Build history of the part. All positions in model axes, mm. A direction names the side the tool comes from. Round coordinates to 2 decimals unless told otherwise and drop trailing zeros. Order: outer loops, then holes, each group sorted by start corner. A loop starts at its lowest first (then second) coordinate and runs counter-clockwise, first axis right, second up. Notation, with made-up numbers: M 38,-24.5 L 62,-24.5 A35 ccw 62,13.5 Z; hole C 6.25,-17 d2. An arc over 180 degrees is marked long. One line per item, written item: value. Start each with the question number.
Item 1: Pin check, flat tips, straight feed: pin 1 (4 mm diameter, centred on y = -2.5, z = 9, fed in from -X); pin 2 (0.8 mm diameter, centred on y = 0, z = 1, fed in from -X); pin 3 (0.8 mm diameter, centred on y = 0, z = 0.5, fed in from +X). Stop position of each tip, or through.
Item 2: Band-saw the part on A-A, the plane z = 10.25. Write the cut outline in (x, y) (3 decimals), then the cut area to 3 significant figures.
Item 3: Band-saw the part on B-B, the plane x = 3. Write the cut outline in (y, z), then the cut area to 3 significant figures.
Item 4: Two-plate mould, pull along Y, no slides. Class faces 5 (the cylindrical face through (1.224, -0.507, 8.52)), 6 (the cylindrical face through (-2.686, -2.06, 2.73)), 7 (the flat face through (-1, -2, 9.78)): +Y half, -Y half, draft (parallel to the pull), parting line (faces both ways), or undercut.
Item 5: Tool access for faces 1 (the flat face through (0, 2.2, 2.35)), 2 (the cylindrical face through (-0.5, -2.4, 12.5)), 3 (the flat face through (0.4, 0, 1)), 4 (the cylindrical face through (0, -2, 6)): list every direction of +Z, -Z, +X, -X, +Y, -Y with a clear straight run to the whole face (end or side of a thin tool).
Item 6: Probe L1, parallel to X at y = 0, z = 8 (3 decimals); L2, parallel to Z at x = 1, y = 0.75; L3, parallel to X at y = 0, z = 11.25 (3 decimals). List the from-to ranges inside material, lowest first.
```python
from build123d import *

# Parameters (mm, degrees)
F0_R      = 3.385
F1_DEPTH  = 15.2
F2_R      = 3.385
F3_DEPTH  = 2.35
F4_DEPTH  = 1.65
F6_R      = 3.385
F6_R_2    = 2.45
F7_DEPTH  = 12.08
F9_R      = 3.385
F9_R_2    = 2
F10_DEPTH = 3
F11_R     = 2.45
F11_R_2   = 2
F12_DEPTH = 0.77
F31_R     = 1.325
F32_DEPTH = 13.55


with BuildPart() as f1:
    # F0 (on Top) → F1 (new body)
    with BuildSketch(Plane.XY):
        Circle(F0_R)
    extrude(amount=F1_DEPTH)

    # F2 (on face) → F3 (cut)
    with BuildSketch(Plane(origin=(0, 0, 0), x_dir=(1, 0, 0), z_dir=(0, 0, -1))):
        Circle(F2_R)
        with BuildLine():
            ThreePointArc((0.4, 1.9595917942), (1.5491933385, 1.2649110641), (2, 0))
            ThreePointArc((2, 0), (1.5491933385, -1.2649110641), (0.4, -1.9595917942))
            ThreePointArc((0.4, -1.9595917942), (0, -2), (-0.4, -1.9595917942))
            ThreePointArc((-0.4, -1.9595917942), (-2, 0), (-0.4, 1.9595917942))
            ThreePointArc((-0.4, 1.9595917942), (0, 2), (0.4, 1.9595917942))
        make_face(mode=Mode.SUBTRACT)
    extrude(amount=-F3_DEPTH, mode=Mode.SUBTRACT)

    # F2 (on face) → F4 (cut)
    with BuildSketch(Plane(origin=(0, 0, 0), x_dir=(1, 0, 0), z_dir=(0, 0, -1))):
        with BuildLine():
            Line((0.4, -1.9595917942), (0.4, 1.9595917942))
            ThreePointArc((0.4, 1.9595917942), (0, 2), (-0.4, 1.9595917942))
            Line((-0.4, 1.9595917942), (-0.4, -1.9595917942))
            ThreePointArc((-0.4, -1.9595917942), (0, -2), (0.4, -1.9595917942))
        make_face()
    extrude(amount=-F4_DEPTH, mode=Mode.SUBTRACT)

    # F6 (on face) → F7 (cut, through all)
    with BuildSketch(Plane.XY.offset(15.2)):
        Circle(F6_R)
        Circle(F6_R_2, mode=Mode.SUBTRACT)
    extrude(amount=-F7_DEPTH, mode=Mode.SUBTRACT)

    # F9 (on offset) → F10 (cut)
    with BuildSketch(Plane.XY.offset(4.5)):
        Circle(F9_R)
        Circle(F9_R_2, mode=Mode.SUBTRACT)
    extrude(amount=F10_DEPTH, mode=Mode.SUBTRACT)

    # F11 (on face) → F12 (cut)
    with BuildSketch(Plane.XY.offset(15.2)):
        Circle(F11_R)
        Circle(F11_R_2, mode=Mode.SUBTRACT)
    extrude(amount=-F12_DEPTH, mode=Mode.SUBTRACT)

    # F20 (on Front) → F28 (revolve, cut)
    with BuildSketch(Plane.XZ):
        Polygon((-2.45, 14.43), (-2.45, 12.875), (-2, 14.43), align=None)
    revolve(axis=Axis((0, 0, 10.2299177088), (0, 0, -1)), mode=Mode.SUBTRACT)

    # F23 (on Front) → F29 (revolve, cut)
    with BuildSketch(Plane.XZ):
        Polygon((-2.45, 12.105), (-2.45, 10.55), (-2, 12.105), align=None)
    revolve(axis=Axis((0, 0, 10.2299177088), (0, 0, -1)), mode=Mode.SUBTRACT)

    # F26 (on Front) → F30 (revolve, cut)
    with BuildSketch(Plane.XZ):
        Polygon((-2.45, 9.78), (-2.45, 8.225), (-2, 9.78), align=None)
    revolve(axis=Axis((0, 0, 10.2299177088), (0, 0, -1)), mode=Mode.SUBTRACT)

    # F31 (on face) → F32 (cut, through all)
    with BuildSketch(Plane.XY.offset(15.2)):
        Circle(F31_R)
    extrude(amount=-F32_DEPTH, mode=Mode.SUBTRACT)


solid = f1.part
```
Output:
1. pin 1: stops at x = -2.36
1. pin 2: stops at x = -2
1. pin 3: stops at x = 2
2. outline: C 0,0 d4.9; hole C 0,0 d2.65
2. area: 13.3 mm²
3. outline: M -1.57,2.35 L 1.57,2.35 L 1.57,3.12 L -1.57,3.12 Z
3. area: 2.41 mm²
4. face 5: undercut
4. face 6: parting line
4. face 7: draft
5. face 1: -Z
5. face 2: +Z
5. face 3: -Z, +Y, -Y
5. face 4: none
6. L1: x = -2.45 to -1.325, 1.325 to 2.45
6. L2: z = 0 to 1.65
6. L3: x = -2.247 to -1.325, 1.325 to 2.247
